```python
from build123d import *

# Parameters (mm, degrees)
SKETCH1_W           = 100
SKETCH1_H           = 40
SKETCH1_R           = 2.2
BOSS_EXTRUDE1_DEPTH = 6


with BuildPart() as part:
    # Sketch1 → Boss-Extrude1 (new body)
    with BuildSketch(Plane.XY.offset(9)):
        with Locations((65, 34)):
            Rectangle(SKETCH1_W, SKETCH1_H)
        with Locations((60, 49)):
            Circle(SKETCH1_R, mode=Mode.SUBTRACT)
        with Locations((20, 19)):
            Circle(SKETCH1_R, mode=Mode.SUBTRACT)
        with Locations((20, 49)):
            Circle(SKETCH1_R, mode=Mode.SUBTRACT)
        with Locations((60, 19)):
            Circle(SKETCH1_R, mode=Mode.SUBTRACT)
    extrude(amount=-BOSS_EXTRUDE1_DEPTH)


solid = part.part
```
Verification items for the finished model (mm, model axes). Coordinates: 2 decimals unless noted, no trailing zeros. Loops run counter-clockwise (first coordinate to the right, second up) from the corner with the lowest first, then second, coordinate; pieces in that order, holes last. Notation, with made-up numbers: (12.25, 28) - (41.25, 28) arc R19 cw to (41.25, 33) - close; hole circle Ø10 at (22, -37.5). An arc over 180 degrees is marked (long way). Answer as a JSON object with one key per item and string values.
(1) Scan lines: line 1 along Y through (x, z) = (60, 4.55); line 2 along X through (y, z) = (19.5, 3.55); line 3 along X through (y, z) = (50, 4.8). Record each from-to range of solid material in increasing order.
Response:
{"line 1": "y = 14 to 16.8, 21.2 to 46.8, 51.2 to 54", "line 2": "x = 15 to 17.86, 22.14 to 57.86, 62.14 to 115", "line 3": "x = 15 to 18.04, 21.96 to 58.04, 61.96 to 115"}
(2) Cross-section at C-C, the plane x = 60. Record the boundary of the cut face in (y, z).
Response:
{"outline": "(14, 3) - (16.8, 3) - (16.8, 9) - (14, 9) - close; (21.2, 3) - (46.8, 3) - (46.8, 9) - (21.2, 9) - close; (51.2, 3) - (54, 3) - (54, 9) - (51.2, 9) - close"}
(3) Go/stop test with a flat-tipped pin: pin 1 Ø2.5 at (x, y) = (20, 49) entering from +Z. Record where the tip stops, or that it passes through.
Response:
{"pin 1": "passes through"}
(4) Cross-section at B-B, the plane y = 19. Record the boundary of the cut face in (x, z), then the cut area to 3 significant figures.
Response:
{"outline": "(15, 3) - (17.8, 3) - (17.8, 9) - (15, 9) - close; (22.2, 3) - (57.8, 3) - (57.8, 9) - (22.2, 9) - close; (62.2, 3) - (115, 3) - (115, 9) - (62.2, 9) - close", "area": "547 mm²"}
(5) Mould release check, pull along X, two halves, no side actions. Record for faces 1 (the flat face through (15, 34, 6)), 2 (the cylindrical face through (62.032, 18.157, 6.042)), 3 (the flat face through (64, 54, 6)): pulls with the +X half, pulls with the -X half, needs draft (parallel to the pull), parting line crosses it, or undercut.
Response:
{"face 1": "pulls with the -X half", "face 2": "undercut", "face 3": "needs draft"}
(6) Cross-section at A-A, the plane z = 7.7. Record the boundary of the cut face in (x, y), then the cut area to 3 significant figures.
Response:
{"outline": "(15, 14) - (115, 14) - (115, 54) - (15, 54) - close; hole circle Ø4.4 at (20, 19); hole circle Ø4.4 at (20, 49); hole circle Ø4.4 at (60, 19); hole circle Ø4.4 at (60, 49)", "area": "3,940 mm²"}
